Could you check a few things on this model? Use its own coordinates, in mm. Round coordinates to 2 decimals unless told otherwise and drop trailing zeros. Loops run counter-clockwise (first coordinate to the right, second up) from the corner with the lowest first, then second, coordinate; pieces in that order, holes last. Notation, with made-up numbers: (41, -15.75) - (96, -15.75) arc R6 cw to (96, -6.75) - close; hole circle Ø8 at (45, 27). An arc over 180 degrees is marked (long way). Put each result on its own line as item: value. Start each with the question number.
Autodesk Inventor part; units mm, degrees
ref_plane "YZ Plane" through (0, 0, 0) normal (1, 0, 0) x (0, 1, 0)
ref_plane "XZ Plane" through (0, 0, 0) normal (0, 1, 0) x (-1, 0, 0)
ref_plane "XY Plane" through (0, 0, 0) normal (0, 0, 1) x (1, 0, 0)
ref_plane "Work Plane1" through (0, 0, 0) normal (0, 0, 1) x (1, 0, 0)
sketch "Sketch1" plane through (0, 0, 0) normal (0, 0, 1) x (1, 0, 0)
  arc A0 (13.0719, -0.4942) -> (13.1202, -0.1498) centre (10.8, 0) ccw
  circle A1 centre (10.8, 0) radius 2.325
  line L0 (10.6, -3.5) -> (10.6, -2.3164)
  line L1 (10.6, -3.5) -> (0, -3.5)
  line L2 (0, -130.1465) -> (0, 181.4158)
  line L3 (10.8, 0) -> (0, 0) construction
  line L4 (10.6, 3.5) -> (10.6, 2.3164)
  line L5 (10.6, 3.5) -> (0, 3.5)
  point P0 (0, 3.5)
  dimension "d1" = 3.5
  dimension "d12" = 4.65
  dimension "d13" = 0.2
  dimension "d14" = 10.8
revolve "Revolution1" add sketch "Sketch1" angle 360 about axis through (0, -130.1465, 0) along (0, 1, 0) contours L0 L1 L2 L5 L4 A1
sketch "Sketch2" plane through (0, 3.5, 0) normal (0, 1, 0) x (1, 0, 0)
  circle A0 centre (4.5, 0) radius 2.2
  circle A1 centre (0, 0) radius 10.6
  circle A2 centre (0, 0) radius 10.6
  circle A3 centre (0, 0) radius 10.6
  circle A4 centre (0, 0) radius 8.35
  circle A5 centre (0, 4.5) radius 2.2
  circle A6 centre (-4.5, 0) radius 2.2
  circle A7 centre (0, -4.5) radius 2.2
  point P0 (0, 0)
  dimension "d3" = 4.4
  dimension "d4" = 2.25
  dimension "d5" = 4.5
  dimension "d8" = 360
extrude "Extrusion1" cut sketch "Sketch2" against normal through all contours A0 | A6
properties part number "Venstre_rotator"
Item 1: Suppose I cut it at A-A, the plane z = 0. List the corners of the cut face in (x, y) for me (3 decimals).
Item 2: Will this pin go through, and if not, where does the flat tip stop? P1, Ø4, axis at x = -4.5, z = 0, coming from the -Y side.
Item 3: Suppose I cut it at D-D, the plane y = 0. List the corners of the cut face in (x, z) for me (3 decimals), then the cut area to 3 significant figures.
Item 4: Thinking about a two-plate mould opening in X: for faces 1 (the face through (0, 3.5, 0)), 2 (the face through (-2.4, 0.05, -0.66)), 3 (the face through (6.6, 0.05, -0.66)), 4 (the face through (9.79, -2.9, 4.06)), which applies, released by +X, released by -X, zero draft, split by the parting line, or undercut?
Item 5: Suppose I cut it at B-B, the plane x = 0. List the corners of the cut face in (y, z) for me (3 decimals), then the cut area to 3 significant figures.
Item 6: Suppose I cut it at C-C, the plane y = -3. List the corners of the cut face in (x, z) for me.
Item 7: I need wall thicknesses on line 1 (X direction, y = 0.5, z = -0.25); line 2 (X direction, y = 1, z = 1.75); line 3 (Z direction, x = -4.5, y = 1.25). Which ranges of each line are inside material? Lowest first, please. Write a range as from..to.
Numbers:
1. outline: (-10.6, -3.5) - (-6.7, -3.5) - (-6.7, 3.5) - (-10.6, 3.5) - (-10.6, 2.316) arc R2.325 cw to (-10.6, -2.316) - close; (-2.3, -3.5) - (2.3, -3.5) - (2.3, 3.5) - (-2.3, 3.5) - close; (6.7, -3.5) - (10.6, -3.5) - (10.6, -2.316) arc R2.325 cw to (10.6, 2.316) - (10.6, 3.5) - (6.7, 3.5) - close
2. P1: through
3. outline: circle Ø16.95 at (0, 0); hole circle Ø4.4 at (-4.5, 0); hole circle Ø4.4 at (4.5, 0)
3. area: 195 mm^2
4. face 1: zero draft
4. face 2: undercut
4. face 3: undercut
4. face 4: split by the parting line
5. outline: (-3.5, -10.6) - (-2.316, -10.6) arc R2.325 cw to (2.316, -10.6) - (3.5, -10.6) - (3.5, 10.6) - (2.316, 10.6) arc R2.325 cw to (-2.316, 10.6) - (-3.5, 10.6) - close
5. area: 133 mm^2
6. outline: circle Ø21.2 at (0, 0); hole circle Ø4.4 at (-4.5, 0); hole circle Ø4.4 at (4.5, 0)
7. line 1: -8.53..-6.69, -2.31..2.31, 6.69..8.53
7. line 2: -8.52..-5.83, -3.17..3.17, 5.83..8.52
7. line 3: -7.61..-2.2, 2.2..7.61
